The listing builds one solid part. Answer for the finished solid, in the listing's coordinates (mm). Coordinates: 2 decimals unless noted, no trailing zeros. Loops run counter-clockwise (first coordinate to the right, second up) from the corner with the lowest first, then second, coordinate; pieces in that order, holes last. Notation, with made-up numbers: (-24.75, 46) - (-19.75, 46) arc R24 ccw to (-19.75, 64) - close; hole circle Ø7 at (28.25, -37). An arc over 180 degrees is marked (long way). Use one line per item in the form item = value. Start each with the question number.
```python
from build123d import *

# Parameters (mm, degrees)
CYLINDER265_R          = 3
CYLINDER265_DEPTH      = 50
CYLINDER265_ROLL_ANGLE = 90
BOX129_W               = 60
BOX129_H               = 22
BOX129_DEPTH           = 23
CYLINDER193_R          = 3
CYLINDER193_DEPTH      = 100
CYLINDER193_ROLL_ANGLE = 90
CYLINDER188_R          = 3
CYLINDER188_DEPTH      = 65
BOX117_W               = 25
BOX117_H               = 15
BOX117_DEPTH           = 15
CYLINDER186_R          = 6
CYLINDER186_DEPTH      = 16
CYLINDER187_R          = 12.5
CYLINDER187_DEPTH      = 4
CYLINDER185_R          = 3
CYLINDER185_DEPTH      = 60
CYLINDER185_ROLL_ANGLE = 90
BOX116_W               = 10
BOX116_H               = 20
BOX116_DEPTH           = 60
CYLINDER184_R          = 14
CYLINDER184_DEPTH      = 320
BOX115_W               = 40
BOX115_H               = 40
BOX115_DEPTH           = 600
CUT233_PLACEMENT_ANGLE = 180


with BuildPart() as obj1:
    # Cylinder265 → Cylinder265 (new body)
    with BuildSketch(Plane.XY):
        Circle(CYLINDER265_R)
    extrude(amount=CYLINDER265_DEPTH)


with BuildPart() as obj1_1:
    # Cylinder265 roll: moved
    add(obj1.part.rotate(Axis((0, 0, 0), (1, 0, 0)), CYLINDER265_ROLL_ANGLE))


with BuildPart() as obj1_2:
    # Cylinder265 placement: moved
    add(obj1_1.part.moved(Location((-466, 485, 211))))


with BuildPart() as cubo092:
    # Box129 → Box129 (new body)
    with BuildSketch(Plane(origin=(-505, 449, 199), x_dir=(1, 0, 0), z_dir=(0, 0, 1))):
        with Locations((30, 11)):
            Rectangle(BOX129_W, BOX129_H)
    extrude(amount=BOX129_DEPTH)


with BuildPart() as obj2:
    # Cylinder193 → Cylinder193 (new body)
    with BuildSketch(Plane.XY):
        Circle(CYLINDER193_R)
    extrude(amount=CYLINDER193_DEPTH)


with BuildPart() as obj2_1:
    # Cylinder193 roll: moved
    add(obj2.part.rotate(Axis((0, 0, 0), (1, 0, 0)), CYLINDER193_ROLL_ANGLE))


with BuildPart() as obj2_2:
    # Cylinder193 placement: moved
    add(obj2_1.part.moved(Location((-450, 50, 211))))


with BuildPart() as cilindro105:
    # Cylinder188 → Cylinder188 (new body)
    with BuildSketch(Plane(origin=(-427.5, 0, -24.5), x_dir=(1, 0, 0), z_dir=(0, 0, 1))):
        Circle(CYLINDER188_R)
    extrude(amount=CYLINDER188_DEPTH)


with BuildPart() as cut236:
    # Box117 → Box117 (new body)
    with BuildSketch(Plane(origin=(-440, -7.5, -8.5), x_dir=(1, 0, 0), z_dir=(0, 0, 1))):
        with Locations((12.5, 7.5)):
            Rectangle(BOX117_W, BOX117_H)
    extrude(amount=BOX117_DEPTH)

    # Cut236: cut Cilindro105
    add(cilindro105.part, mode=Mode.SUBTRACT)


with BuildPart() as obj3:
    # Cylinder186 → Cylinder186 (new body)
    with BuildSketch(Plane(origin=(-460, 0, -11), x_dir=(1, 0, 0), z_dir=(0, 0, 1))):
        Circle(CYLINDER186_R)
    extrude(amount=CYLINDER186_DEPTH)


with BuildPart() as rodamiento006:
    # Cylinder187 → Cylinder187 (new body)
    with BuildSketch(Plane(origin=(-460, 0, -15), x_dir=(1, 0, 0), z_dir=(0, 0, 1))):
        Circle(CYLINDER187_R)
    extrude(amount=CYLINDER187_DEPTH)


with BuildPart() as obj4:
    # Sphere017 → Sphere017 (revolve)
    with BuildSketch(Plane(origin=(8, 0, 265), x_dir=(1, 0, 0), z_dir=(0, -1, 0))):
        with BuildLine():
            ThreePointArc((0, -14), (14, 0), (0, 14))
            Line((0, 14), (0, -14))
        make_face()
    revolve(axis=Axis((8, 0, 265), (0, 0, 1)))


with BuildPart() as obj5:
    # Cylinder185 → Cylinder185 (new body)
    with BuildSketch(Plane.XY):
        Circle(CYLINDER185_R)
    extrude(amount=CYLINDER185_DEPTH)


with BuildPart() as obj5_1:
    # Cylinder185 roll: moved
    add(obj5.part.rotate(Axis((0, 0, 0), (1, 0, 0)), CYLINDER185_ROLL_ANGLE))


with BuildPart() as obj5_2:
    # Cylinder185 placement: moved
    add(obj5_1.part.moved(Location((32, 30, 532))))


with BuildPart() as obj6:
    # Box116 → Box116 (new body)
    with BuildSketch(Plane(origin=(27, -10, 525), x_dir=(1, 0, 0), z_dir=(0, 0, 1))):
        with Locations((5, 10)):
            Rectangle(BOX116_W, BOX116_H)
    extrude(amount=BOX116_DEPTH)


with BuildPart() as obj7:
    # Cylinder184 → Cylinder184 (new body)
    with BuildSketch(Plane(origin=(8, 0, 265), x_dir=(1, 0, 0), z_dir=(0, 0, 1))):
        Circle(CYLINDER184_R)
    extrude(amount=CYLINDER184_DEPTH)


with BuildPart() as cut285:
    # Box115 → Box115 (new body)
    with BuildSketch(Plane(origin=(0, -20, -15), x_dir=(1, 0, 0), z_dir=(0, 0, 1))):
        with Locations((20, 20)):
            Rectangle(BOX115_W, BOX115_H)
    extrude(amount=BOX115_DEPTH)

    # Cut230: cut obj7
    add(obj7.part, mode=Mode.SUBTRACT)

    # Cut231: cut obj6
    add(obj6.part, mode=Mode.SUBTRACT)

    # Cut232: cut obj5
    add(obj5_2.part, mode=Mode.SUBTRACT)

    # Cut233: cut obj4
    add(obj4.part, mode=Mode.SUBTRACT)


with BuildPart() as cut285_1:
    # Cut233 placement: moved
    add(cut285.part.moved(Location((-440, 0, 0))).rotate(Axis((-440, 0, 0), (0, 0, 1)), CUT233_PLACEMENT_ANGLE))

    # Cut234: cut rodamiento006
    add(rodamiento006.part, mode=Mode.SUBTRACT)

    # Cut235: cut obj3
    add(obj3.part, mode=Mode.SUBTRACT)

    # Fusion057: union Cut236
    add(cut236.part)

    # Cut244: cut obj2
    add(obj2_2.part, mode=Mode.SUBTRACT)


with BuildPart() as cut285_2:
    # Cut244 placement: moved
    add(cut285_1.part.moved(Location((0, 460, 0))))

    # Cut284: cut Cubo092
    add(cubo092.part, mode=Mode.SUBTRACT)

    # Cut285: cut obj1
    add(obj1_2.part, mode=Mode.SUBTRACT)


solid = cut285_2.part
```
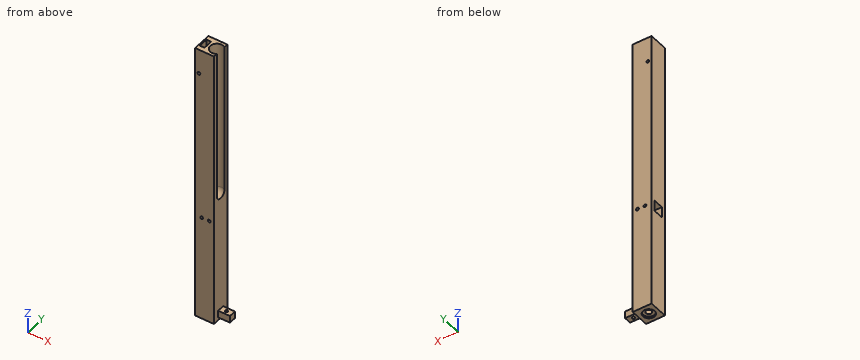
(1) Each of these flat-tipped pins is pushed along its axis until it touches: pin 1 Ø11 at (y, z) = (461.5, 215.5) entering from -X; pin 2 Ø7.5 at (x, y) = (-464, 456) entering from -Z; pin 3 Ø3.5 at (x, y) = (-461, 459) entering from -Z. Where does it stop, or does it pass through?
(2) A cutting plane is placed at B-B (z = 30). Determine the outline of the cut face in (x, y).
(3) Find the intervals of material crossed by probe 1 along X at (y, z) = (460, 0); probe 2 along X at (y, z) = (473.75, 211); probe 3 along Y at (x, z) = (-448, 458.5), in increasing order. Write a range as from..to.
(4) A cutting plane is placed at A-A (z = 355). Determine the outline of the cut face in (x, y), then the cut area to 3 significant figures.
Evaluation:
q1.pin_1 = -445
q1.pin_2 = -11
q1.pin_3 = 5
q2.outline = (-480, 440) - (-440, 440) - (-440, 480) - (-480, 480) - close
q3.probe_1 = -480..-466, -454..-430.5, -424.5..-415
q3.probe_2 = -480..-469, -463..-453, -447..-440
q3.probe_3 = 440..446, 474..480
q4.outline = (-480, 440) - (-440, 440) - (-440, 448.51) arc R14 cw (long way) to (-440, 471.49) - (-440, 480) - (-480, 480) - close
q4.area = 1,080 mm^2
